from build123d import *

# Parameters (mm, degrees)
F0_W     = 13.589
F0_H     = 8.382
F0_R     = 2.159
F1_DEPTH = 9.144
F2_W     = 13.589
F2_H     = 8.382
F2_R     = 2.159
F2_R_2   = 1.143
F3_DEPTH = 5.08
F4_W     = 16.764
F4_H     = 11.557
F4_W_2   = 13.589
F4_H_2   = 8.382
F4_R     = 1.143
F5_DEPTH = 8.89
F6_SIZE  = 0.635
F7_W     = 16.764
F7_H     = 11.557
F7_W_2   = 13.589
F7_H_2   = 8.382
F8_DEPTH = 3.81


with BuildPart() as f1:
    # F0 (on Top) → F1 (new body)
    with BuildSketch(Plane.XY):
        Rectangle(F0_W, F0_H)
        with Locations((-3.81, 0)):
            Circle(F0_R, mode=Mode.SUBTRACT)
        with Locations((3.81, 0)):
            Circle(F0_R, mode=Mode.SUBTRACT)
    extrude(amount=F1_DEPTH)

    # F2 (on face) → F3 (join)
    with BuildSketch(Plane.XY.offset(9.144)):
        Rectangle(F2_W, F2_H)
        with Locations((-3.81, 0)):
            Circle(F2_R, mode=Mode.SUBTRACT)
        with Locations((3.81, 0)):
            Circle(F2_R, mode=Mode.SUBTRACT)
        with Locations((-3.81, 0)):
            Circle(F2_R)
        with Locations((-3.81, 0)):
            Circle(F2_R_2, mode=Mode.SUBTRACT)
        with Locations((3.81, 0)):
            Circle(F2_R)
        with Locations((3.81, 0)):
            Circle(F2_R_2, mode=Mode.SUBTRACT)
    extrude(amount=F3_DEPTH)

    # F4 (on face) → F5 (join)
    with BuildSketch(Plane.XY.offset(14.224)):
        Rectangle(F4_W, F4_H)
        Rectangle(F4_W_2, F4_H_2, mode=Mode.SUBTRACT)
        Rectangle(F4_W_2, F4_H_2)
        with Locations((-3.81, 0)):
            Circle(F4_R, mode=Mode.SUBTRACT)
        with Locations((3.81, 0)):
            Circle(F4_R, mode=Mode.SUBTRACT)
    extrude(amount=F5_DEPTH)

    # F6
    f6_edges = [f1.edges().sort_by_distance(p)[0] for p in [
        (-6.7945, 4.191, 7.112),
        (-6.7945, -4.191, 7.112),
        (6.7945, 4.191, 7.112),
        (6.7945, -4.191, 7.112),
    ]]
    chamfer(f6_edges, length=F6_SIZE)

    # F7 (on face) → F8 (join)
    with BuildSketch(Plane.XY.offset(23.114)):
        Rectangle(F7_W, F7_H)
        Rectangle(F7_W_2, F7_H_2, mode=Mode.SUBTRACT)
    extrude(amount=F8_DEPTH)


solid = f1.part
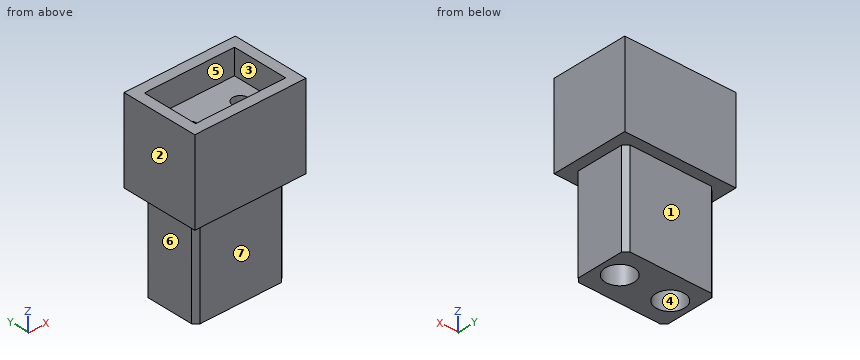
Build history of the part. All positions in model axes, mm. Face numbers are marked on the shaded views. A direction names the side the tool comes from. Round coordinates to 2 decimals unless told otherwise and drop trailing zeros. Write each loop counter-clockwise with the first axis right and the second up, starting at its lowest first coordinate (ties: lowest second). Pieces come first, ordered by that corner, then holes. Notation, with made-up numbers: M 1,17 L 50,17 A12 cw 50,35 Z; hole C 77.25,35 d8. An arc over 180 degrees is marked long. Use CSV: the item, a comma, the result in double quotes.
1. Saw through at A-A (y = 0). Give the cut face in (x, z).
Reply:
outline,"M -8.38,14.22 L -6.79,14.22 L -6.79,0 L -5.97,0 L -5.97,9.14 L -4.95,9.14 L -4.95,23.11 L -6.79,23.11 L -6.79,26.92 L -8.38,26.92 Z; M -2.67,9.14 L -1.65,9.14 L -1.65,0 L 1.65,0 L 1.65,9.14 L 2.67,9.14 L 2.67,23.11 L -2.67,23.11 Z; M 4.95,9.14 L 5.97,9.14 L 5.97,0 L 6.79,0 L 6.79,14.22 L 8.38,14.22 L 8.38,26.92 L 6.79,26.92 L 6.79,23.11 L 4.95,23.11 Z"
2. Tool access for the marked faces 5, 6 and 7: list every direction of +Z, -Z, +X, -X, +Y, -Y with a clear straight run to the whole face (end or side of a thin tool).
Reply:
face 5,"+Z"
face 6,"-Z, -X, +Y, -Y"
face 7,"-Z, +X, -X, -Y"
3. Flat gauge pins, fed straight in: pin 1 (1.5 mm diameter, centred on x = 5.5, y = 0.5, fed in from -Z); pin 2 (6.5 mm diameter, centred on x = -3.5, y = 0, fed in from +Z); pin 3 (3.5 mm diameter, centred on x = -3.81, y = 0, fed in from -Z); pin 4 (2 mm diameter, centred on y = -0.5, z = 9.5, fed in from -X). Where does each tip first touch, or does it go through?
Reply:
pin 1,"stops at z = 0"
pin 2,"stops at z = 23.11"
pin 3,"stops at z = 9.14"
pin 4,"stops at x = -6.79"
4. Saw through at C-C (z = 3). Give the cut face in (x, y), plus the area to 3 significant figures.
Reply:
outline,"M -6.79,-3.56 L -6.16,-4.19 L 6.16,-4.19 L 6.79,-3.56 L 6.79,3.56 L 6.16,4.19 L -6.16,4.19 L -6.79,3.56 Z; hole C -3.81,0 d4.32; hole C 3.81,0 d4.32"
area,"83.8 mm²"
5. Saw through at B-B (x = 3.81). Give the cut face in (y, z), plus the area to 3 significant figures.
Reply:
outline,"M -5.78,14.22 L -4.19,14.22 L -4.19,0 L -2.16,0 L -2.16,9.14 L -1.14,9.14 L -1.14,23.11 L -4.19,23.11 L -4.19,26.92 L -5.78,26.92 Z; M 1.14,9.14 L 2.16,9.14 L 2.16,0 L 4.19,0 L 4.19,14.22 L 5.78,14.22 L 5.78,26.92 L 4.19,26.92 L 4.19,23.11 L 1.14,23.11 Z"
area,"163 mm²"
6. Two-plate mould, pull along X, no slides. Class the marked faces 1, 2, 3 and 4: +X half, -X half, draft (parallel to the pull), parting line (faces both ways), or undercut.
Reply:
face 1,"draft"
face 2,"-X half"
face 3,"undercut"
face 4,"undercut"
7. Wall check: probe 1 along Y at (x, z) = (3.81, 2); probe 2 along X at (y, z) = (-1.5, 3); probe 3 along Y at (x, z) = (3.81, 17). Give the ranges that are in metal, low to high. Write a range as from..to.
Reply:
probe 1,"y = -4.19..-2.16, 2.16..4.19"
probe 2,"x = -6.79..-5.36, -2.26..2.26, 5.36..6.79"
probe 3,"y = -5.78..-1.14, 1.14..5.78"
8. Saw through at D-D (y = 3). Give the cut face in (x, z), plus the area to 3 significant figures.
Reply:
outline,"M -8.38,14.22 L -6.79,14.22 L -6.79,0 L 6.79,0 L 6.79,14.22 L 8.38,14.22 L 8.38,26.92 L 6.79,26.92 L 6.79,23.11 L -6.79,23.11 L -6.79,26.92 L -8.38,26.92 Z"
area,"354 mm²"
